from build123d import *

# Parameters (mm, degrees)
CYLINDER001_R     = 1.5
CYLINDER001_DEPTH = 20
ARRAY_COUNT       = 8
CYLINDER_R        = 10
CYLINDER_DEPTH    = 15


with BuildPart() as array:
    # Cylinder001 → Cylinder001 (new body)
    with BuildSketch(Plane(origin=(10.5, 0, -2), x_dir=(1, 0, 0), z_dir=(0, 0, 1))):
        Circle(CYLINDER001_R)
    extrude(amount=CYLINDER001_DEPTH)

    # Array: Array ×8 about axis
    array_axis = Axis((0, 0, 1), (0, 0, 1))


with BuildPart() as array_1:
    add(array.part)
    for i in range(1, ARRAY_COUNT):
        add(array.part.rotate(array_axis, i * 360 / ARRAY_COUNT))


with BuildPart() as obj1:
    # Cylinder → Cylinder (new body)
    with BuildSketch(Plane.XY):
        Circle(CYLINDER_R)
    extrude(amount=CYLINDER_DEPTH)

    # Cut: cut Array
    add(array_1.part, mode=Mode.SUBTRACT)


solid = obj1.part
Work out the finished part from the listing and answer in its coordinate system (mm). Round coordinates to 2 decimals unless told otherwise and drop trailing zeros. Write each loop counter-clockwise with the first axis right and the second up, starting at its lowest first coordinate (ties: lowest second). Pieces come first, ordered by that corner, then holes. Notation, with made-up numbers: (68, 71.5) -> (108, 71.5) arc R29 ccw to (108, 91.5) -> close; hole circle Ø3 at (-16, 58). An arc over 180 degrees is marked (long way). Write each question's results on one line, items separated by ' | '.
Item 1: Find the intervals of material crossed by line 1 along Y through (x, z) = (-7.5, 9.5); line 2 along Y through (x, z) = (-5.5, 11.5); line 3 along X through (y, z) = (3.5, 8), in increasing order. Write a range as [from, to].
Result set:
line 1: [-5.93, 5.93] | line 2: [-8.35, 8.35] | line 3: [-9.37, 9.37]
Item 2: A cutting plane is placed at A-A, the plane z = 4.5. Determine the outline of the cut face in (x, y), plus the area to 3 significant figures.
Result set:
outline: (-9.9, -1.38) arc R10 ccw to (-7.98, -6.03) arc R1.5 cw to (-6.03, -7.98) arc R10 ccw to (-1.38, -9.9) arc R1.5 cw to (1.38, -9.9) arc R10 ccw to (6.03, -7.98) arc R1.5 cw to (7.98, -6.03) arc R10 ccw to (9.9, -1.38) arc R1.5 cw to (9.9, 1.38) arc R10 ccw to (7.98, 6.03) arc R1.5 cw to (6.03, 7.98) arc R10 ccw to (1.38, 9.9) arc R1.5 cw to (-1.38, 9.9) arc R10 ccw to (-6.03, 7.98) arc R1.5 cw to (-7.98, 6.03) arc R10 ccw to (-9.9, 1.38) arc R1.5 cw to start | area: 298 mm^2
Item 3: A cutting plane is placed at B-B, the plane x = -8.5. Determine the outline of the cut face in (y, z), plus the area to 3 significant figures.
Result set:
outline: (-5.27, 0) -> (5.27, 0) -> (5.27, 15) -> (-5.27, 15) -> close | area: 158 mm^2
Item 4: The mould has two halves that part along Y. Classify faces 1 (the face through (-3.794, 9.252, 7.395)), 2 (the face through (0, 0, 0)), 3 (the face through (-9, 0, 7)): +Y half, -Y half, draft (parallel to the pull), parting line (faces both ways), or undercut.
Result set:
face 1: +Y half | face 2: draft | face 3: undercut
Item 5: A cutting plane is placed at C-C, the plane y = -6.75. Determine the outline of the cut face in (x, z), plus the area to 3 significant figures.
Result set:
outline: (-6.08, 0) -> (6.08, 0) -> (6.08, 15) -> (-6.08, 15) -> close | area: 183 mm^2
Item 6: Flat-ended cylindrical pins translate along their axes: P1, Ø1, axis at x = 0.5, z = 11.5, coming from the -Y side; P2, Ø2, axis at y = 5, z = 3.5, coming from the -X side. Find the tip coordinate at first contact, or state that the pin passes through.
Result set:
P1: y = -9.38 | P2: x = -9.17
